Here's how the part is built. I have some questions about the finished solid (model axes, mm). A direction names the side the tool comes from. Round coordinates to 2 decimals unless told otherwise and drop trailing zeros. Order: outer loops, then holes, each group sorted by start corner. A loop starts at its lowest first (then second) coordinate and runs counter-clockwise, first axis right, second up. Notation, with made-up numbers: (-1, 88.25) - (23, 88.25) arc R30 cw to (23, 119.25) - close; hole circle Ø9 at (72, -39). An arc over 180 degrees is marked (long way). One line per item, written item: value.
from build123d import *

# Parameters (mm, degrees)
SKETCH1_W           = 36.5
SKETCH1_H           = 27
BOSS_EXTRUDE1_DEPTH = 2
BOSS_EXTRUDE2_DEPTH = 1.7
CUT_EXTRUDE1_REACH  = 24.788
FILL_PATTERN1_DEPTH = 2
CUT_EXTRUDE3_REACH  = 25
SKETCH5_W           = 0.75
SKETCH5_H           = 2.2
SKETCH6_W           = 11.033121635
SKETCH6_H           = 27
CUT_EXTRUDE4_DEPTH  = 24.000054348


# Read off the part's stored shape, not the designer's step: Fill Pattern1
with BuildPart() as part:
    # Sketch1 → Boss-Extrude1 (new body)
    with BuildSketch(Plane.XY):
        Rectangle(SKETCH1_W, SKETCH1_H)
    extrude(amount=BOSS_EXTRUDE1_DEPTH)

    # Sketch2 → Boss-Extrude2 (add)
    with BuildSketch(Plane(origin=(0, 0, 0), x_dir=(-1, 0, 0), z_dir=(0, 0, -1))):
        Polygon((-17.4, 12.3), (-16.6, 12.3), (-16.6, -11.85), (0, -11.85), (0, -12.65), (-17.4, -12.65), align=None)
    boss_extrude2 = extrude(amount=BOSS_EXTRUDE2_DEPTH)

    # Mirror1: Boss-Extrude2 across plane
    add(boss_extrude2.mirror(Plane(origin=(0, 0, 0), x_dir=(0, 0, 1), z_dir=(1, 0, 0))))

    # Sketch3 → Cut-Extrude1 (cut, up to next)
    with BuildSketch(Plane(origin=(0, 0, 0), x_dir=(-1, 0, 0), z_dir=(0, 0, -1)), mode=Mode.PRIVATE) as cut_extrude1_sk1:
        Polygon((-1.154700538, 2), (-2.309401077, 0), (-1.154700538, -2), (1.154700538, -2), (2.309401077, 0), (1.154700538, 2), align=None)
    cut_extrude1_tool1 = extrude(cut_extrude1_sk1.sketch, amount=-CUT_EXTRUDE1_REACH, mode=Mode.PRIVATE) & part.part
    add(cut_extrude1_tool1.solids().sort_by_distance((0, 0, 0))[0], mode=Mode.SUBTRACT)

    # Fill Pattern1 outline → Fill Pattern1 (cut)
    with BuildSketch(Plane.XY):
        Polygon((11.835680518, 0), (10.68097998, 2), (8.371578903, 2), (7.216878365, 0), (8.371578903, -2), (10.68097998, -2), align=None)
        Polygon((-7.216878365, 0), (-8.371578903, 2), (-10.68097998, 2), (-11.835680518, 0), (-10.68097998, -2), (-8.371578903, -2), align=None)
        Polygon((-3.608439182, -6.25), (-5.917840259, -6.25), (-7.072540798, -8.25), (-5.917840259, -10.25), (-3.608439182, -10.25), (-2.453738644, -8.25), align=None)
        Polygon((5.917840259, 10.25), (3.608439182, 10.25), (2.453738644, 8.25), (3.608439182, 6.25), (5.917840259, 6.25), (7.072540798, 8.25), align=None)
        Polygon((-5.917840259, 10.25), (-7.072540798, 8.25), (-5.917840259, 6.25), (-3.608439182, 6.25), (-2.453738644, 8.25), (-3.608439182, 10.25), align=None)
        Polygon((3.608439182, -6.25), (2.453738644, -8.25), (3.608439182, -10.25), (5.917840259, -10.25), (7.072540798, -8.25), (5.917840259, -6.25), align=None)
        Polygon((2.309401077, 5.5), (1.154700538, 7.5), (-1.154700538, 7.5), (-2.309401077, 5.5), (-1.154700538, 3.5), (1.154700538, 3.5), align=None)
        Polygon((-7.216878365, 5.5), (-8.371578903, 7.5), (-10.68097998, 7.5), (-11.835680518, 5.5), (-10.68097998, 3.5), (-8.371578903, 3.5), align=None)
        Polygon((11.835680518, 5.5), (10.68097998, 7.5), (8.371578903, 7.5), (7.216878365, 5.5), (8.371578903, 3.5), (10.68097998, 3.5), align=None)
        Polygon((-3.608439182, -0.75), (-5.917840259, -0.75), (-7.072540798, -2.75), (-5.917840259, -4.75), (-3.608439182, -4.75), (-2.453738644, -2.75), align=None)
        Polygon((3.608439182, -0.75), (2.453738644, -2.75), (3.608439182, -4.75), (5.917840259, -4.75), (7.072540798, -2.75), (5.917840259, -0.75), align=None)
        Polygon((7.072540798, 2.75), (5.917840259, 4.75), (3.608439182, 4.75), (2.453738644, 2.75), (3.608439182, 0.75), (5.917840259, 0.75), align=None)
        Polygon((-2.453738644, 2.75), (-3.608439182, 4.75), (-5.917840259, 4.75), (-7.072540798, 2.75), (-5.917840259, 0.75), (-3.608439182, 0.75), align=None)
        Polygon((1.154700538, -3.5), (-1.154700538, -3.5), (-2.309401077, -5.5), (-1.154700538, -7.5), (1.154700538, -7.5), (2.309401077, -5.5), align=None)
        Polygon((8.371578903, -3.5), (7.216878365, -5.5), (8.371578903, -7.5), (10.68097998, -7.5), (11.835680518, -5.5), (10.68097998, -3.5), align=None)
        Polygon((-7.216878365, -5.5), (-8.371578903, -3.5), (-10.68097998, -3.5), (-11.835680518, -5.5), (-10.68097998, -7.5), (-8.371578903, -7.5), align=None)
    extrude(amount=FILL_PATTERN1_DEPTH, mode=Mode.SUBTRACT)

    # Sketch5 → Cut-Extrude3 (cut, up to next)
    with BuildSketch(Plane.XY.offset(2), mode=Mode.PRIVATE) as cut_extrude3_sk1:
        with Locations((17.875, -4.1)):
            Rectangle(SKETCH5_W, SKETCH5_H)
    cut_extrude3_tool1 = extrude(cut_extrude3_sk1.sketch, amount=-CUT_EXTRUDE3_REACH, mode=Mode.PRIVATE) & part.part
    cut_extrude3 = cut_extrude3_tool1.solids().sort_by_distance((17.875, -4.1, 2))[0]
    add(cut_extrude3, mode=Mode.SUBTRACT)

    # Mirror2: Cut-Extrude3 across plane
    add(cut_extrude3.mirror(Plane(origin=(0, 0, 0), x_dir=(0, 0, 1), z_dir=(1, 0, 0))), mode=Mode.SUBTRACT)

    # Sketch6 → Cut-Extrude4 (cut, through all)
    with BuildSketch(Plane.XY.offset(2)):
        with Locations((-12.733439182, 0)):
            Rectangle(SKETCH6_W, SKETCH6_H)
    extrude(amount=-CUT_EXTRUDE4_DEPTH, mode=Mode.SUBTRACT)


solid = part.part
Q1. If I drill on line 1 along Y through (x, z) = (4, 0.15); line 2 along Y through (x, z) = (10.5, 1.25); line 3 along X through (y, z) = (-2.25, 1.8), over which ranges is the centre line in solid material (lowest first)?
Results list:
line 1: -13.5 to -10.25, -6.25 to -4.75, -0.75 to 0.75, 4.75 to 6.25, 10.25 to 13.5
line 2: -13.5 to -7.5, -3.5 to -2, 2 to 3.5, 7.5 to 13.5
line 3: -7.22 to -6.78, -2.74 to 2.74, 6.78 to 18.25
Q2. If we section it at A-A, the plane x = -0.5: Please give me the cut outline in (y, z).
Results list:
outline: (-13.5, 0) - (-12.65, 0) - (-12.65, -1.7) - (-11.85, -1.7) - (-11.85, 0) - (-7.5, 0) - (-7.5, 2) - (-13.5, 2) - close; (-3.5, 0) - (-2, 0) - (-2, 2) - (-3.5, 2) - close; (2, 0) - (3.5, 0) - (3.5, 2) - (2, 2) - close; (7.5, 0) - (13.5, 0) - (13.5, 2) - (7.5, 2) - close
Q3. Will these pins go through, and if not, where does the flat tip stop? pin 1 (7.5 mm diameter, centred on x = 10, y = -1, fed in from -Z); pin 2 (0.8 mm diameter, centred on y = -3.5, z = -0.5, fed in from -X); pin 3 (0.8 mm diameter, centred on x = 7.5, z = -1, fed in from -Y).
Results list:
pin 1: z = 0
pin 2: x = 16.6
pin 3: y = -12.65
Q4. We'd pull the mould along Y, two halves only. Please class faces 4 (the flat face through (5, -12.65, -1)), 5 (the flat face through (17, -6, -1.7)), 6 (the flat face through (6.5, 3.74, 0.99)): released by +Y, released by -Y, zero draft, split by the parting line, or undercut.
Results list:
face 4: released by -Y
face 5: zero draft
face 6: undercut
Q5. If we section it at C-C, the plane z = -0.8: Please give me the cut outline in (x, y), then the cut area to 3 significant figures.
Results list:
outline: (-7.22, -12.65) - (17.4, -12.65) - (17.4, 12.3) - (16.6, 12.3) - (16.6, -11.85) - (-7.22, -11.85) - close
area: 39.0 mm²
Q6. If we section it at B-B, the plane x = -5: Please give me the cut outline in (y, z).
Results list:
outline: (-13.5, 0) - (-12.65, 0) - (-12.65, -1.7) - (-11.85, -1.7) - (-11.85, 0) - (-10.25, 0) - (-10.25, 2) - (-13.5, 2) - close; (-6.25, 0) - (-4.75, 0) - (-4.75, 2) - (-6.25, 2) - close; (-0.75, 0) - (0.75, 0) - (0.75, 2) - (-0.75, 2) - close; (4.75, 0) - (6.25, 0) - (6.25, 2) - (4.75, 2) - close; (10.25, 0) - (13.5, 0) - (13.5, 2) - (10.25, 2) - close
Q7. Which directions (+Z, -Z, +X, -X, +Y, -Y) give clear straight access to the entire face, cutting with the end or side of a thin tool? Please do faces 1 (the flat face through (5, 0, 2)), 2 (the flat face through (17.4, 0, -1)), 3 (the flat face through (-5, 10.25, 1)).
Results list:
face 1: +Z, +X, -X, +Y, -Y
face 2: -Z, +X, +Y, -Y
face 3: +Z, -Z
Q8. If we section it at D-D, the plane y = 9: Please give me the cut outline in (x, z), then the cut area to 3 significant figures.
Results list:
outline: (-7.22, 0) - (-6.64, 0) - (-6.64, 2) - (-7.22, 2) - close; (-2.89, 0) - (2.89, 0) - (2.89, 2) - (-2.89, 2) - close; (6.64, 0) - (16.6, 0) - (16.6, -1.7) - (17.4, -1.7) - (17.4, 0) - (18.25, 0) - (18.25, 2) - (6.64, 2) - close
area: 37.3 mm²
